from build123d import *

# Parameters (mm, degrees)
ESBO_O1_W                = 49.1
ESBO_O1_H                = 29.84
ESBO_O1_R                = 5.05
RESSALTO_EXTRUS_O1_DEPTH = 1.8
ESBO_O2_W                = 42
ESBO_O2_H                = 29.84
ESBO_O2_R                = 1.35
RESSALTO_EXTRUS_O2_DEPTH = 1.8
RESSALTO_EXTRUS_O3_START = 1.8
ESBO_O3_W                = 42
ESBO_O3_H                = 29.84
ESBO_O3_R                = 1.35
RESSALTO_EXTRUS_O3_DEPTH = 1.8


with BuildPart() as part:
    # Esboço1 → Ressalto-extrusão1 (new body)
    with BuildSketch(Plane.XY):
        Rectangle(ESBO_O1_W, ESBO_O1_H)
        Circle(ESBO_O1_R, mode=Mode.SUBTRACT)
    extrude(amount=RESSALTO_EXTRUS_O1_DEPTH)

    # Esboço2 → Ressalto-extrusão2 (add)
    with BuildSketch(Plane.ZY.offset(24.55)):
        with Locations((21, 0)):
            Rectangle(ESBO_O2_W, ESBO_O2_H)
        with Locations((32, 0)):
            Circle(ESBO_O2_R, mode=Mode.SUBTRACT)
        with Locations((25.05, 7)):
            Circle(ESBO_O2_R, mode=Mode.SUBTRACT)
        with Locations(Location((18, 0, 0), (0, 0, 180))):
            Circle(ESBO_O2_R, mode=Mode.SUBTRACT)
        with Locations(Location((25.05, -7, 0), (0, 0, 180))):
            Circle(ESBO_O2_R, mode=Mode.SUBTRACT)
    extrude(amount=RESSALTO_EXTRUS_O2_DEPTH)

    # Esboço3 → Ressalto-extrusão3 (add)
    with BuildSketch(Plane(origin=(24.55, 0, 0), x_dir=(0, 0, -1), z_dir=(1, 0, 0)).offset(RESSALTO_EXTRUS_O3_START)):
        with Locations((-21, 0)):
            Rectangle(ESBO_O3_W, ESBO_O3_H)
        with Locations(Location((-25.05, 7, 0), (0, 0, 180))):
            Circle(ESBO_O3_R, mode=Mode.SUBTRACT)
        with Locations((-18, 0)):
            Circle(ESBO_O3_R, mode=Mode.SUBTRACT)
        with Locations(Location((-32, 0, 0), (0, 0, 180))):
            Circle(ESBO_O3_R, mode=Mode.SUBTRACT)
        with Locations((-25.05, -7)):
            Circle(ESBO_O3_R, mode=Mode.SUBTRACT)
    extrude(amount=-RESSALTO_EXTRUS_O3_DEPTH)


solid = part.part
Input: part model. Units: mm. Frame: model coordinates. A direction names the side the tool comes from. Coordinates: 2 decimals unless noted, no trailing zeros. Loops run counter-clockwise (first coordinate to the right, second up) from the corner with the lowest first, then second, coordinate; pieces in that order, holes last. Notation, with made-up numbers: (32.25, -39.5) -> (78.25, -39.5) arc R14 ccw to (78.25, -30.5) -> close; hole circle Ø3 at (89.25, 67.25). An arc over 180 degrees is marked (long way). One line per item, written item: value.
(1) Ray query, line 1 along Y through (x, z) = (-25.1, 25.05); line 2 along Y through (x, z) = (25.95, 32); line 3 along X through (y, z) = (-8, 23.5). Return the intervals inside material, ascending.
Answer below:
line 1: y = -14.92 to -8.35, -5.65 to 5.65, 8.35 to 14.92
line 2: y = -14.92 to -1.35, 1.35 to 14.92
line 3: x = -26.35 to -24.55, 24.55 to 26.35
(2) Set-up query: faces 4 (the face through (25, 0, 42)), 5 (the face through (-24.55, 0, 22)). Return all of +Z, -Z, +X, -X, +Y, -Y with unobstructed straight access to the full face (end or side cutting, diameter ignored); none if empty.
Answer below:
face 4: +Z, +X, -X, +Y, -Y
face 5: +Z, +Y, -Y
(3) Cut plane B-B (y = -7). Output: boundary loops of the cut face in (x, z), then the cut area to 3 significant figures.
Answer below:
outline: (-26.35, 0) -> (26.35, 0) -> (26.35, 23.7) -> (24.55, 23.7) -> (24.55, 1.8) -> (-24.55, 1.8) -> (-24.55, 23.7) -> (-26.35, 23.7) -> close; (-26.35, 26.4) -> (-24.55, 26.4) -> (-24.55, 42) -> (-26.35, 42) -> close; (24.55, 26.4) -> (26.35, 26.4) -> (26.35, 42) -> (24.55, 42) -> close
area: 230 mm2
(4) Cut plane A-A (x = 0). Output: boundary loops of the cut face in (y, z), then the cut area to 3 significant figures.
Answer below:
outline: (-14.92, 0) -> (-5.05, 0) -> (-5.05, 1.8) -> (-14.92, 1.8) -> close; (5.05, 0) -> (14.92, 0) -> (14.92, 1.8) -> (5.05, 1.8) -> close
area: 35.5 mm2
(5) Cut plane D-D (y = 0). Output: boundary loops of the cut face in (x, z).
Answer below:
outline: (-26.35, 0) -> (-5.05, 0) -> (-5.05, 1.8) -> (-24.55, 1.8) -> (-24.55, 16.65) -> (-26.35, 16.65) -> close; (-26.35, 19.35) -> (-24.55, 19.35) -> (-24.55, 30.65) -> (-26.35, 30.65) -> close; (-26.35, 33.35) -> (-24.55, 33.35) -> (-24.55, 42) -> (-26.35, 42) -> close; (5.05, 0) -> (26.35, 0) -> (26.35, 16.65) -> (24.55, 16.65) -> (24.55, 1.8) -> (5.05, 1.8) -> close; (24.55, 19.35) -> (26.35, 19.35) -> (26.35, 30.65) -> (24.55, 30.65) -> close; (24.55, 33.35) -> (26.35, 33.35) -> (26.35, 42) -> (24.55, 42) -> close
(6) Pin query (flat end, axial travel): pin 1 Ø3 at (x, y) = (0, -11.5) entering from -Z; pin 2 Ø11.5 at (x, y) = (0, 0) entering from +Z. Return the tip coordinate at first contact, or that it passes through.
Answer below:
pin 1: stops at z = 0
pin 2: stops at z = 1.8
(7) Draft query along X for faces 1 (the face through (-6, 0, 1.8)), 2 (the face through (0, -14.92, 1)), 3 (the face through (-26.35, 0, 21)). Return one class per face: pulls with the +X half, pulls with the -X half, needs draft (parallel to the pull), parting line crosses it, or undercut.
Answer below:
face 1: undercut
face 2: needs draft
face 3: pulls with the -X half
(8) Cut plane C-C (z = 18). Output: boundary loops of the cut face in (x, y).
Answer below:
outline: (-26.35, -14.92) -> (-24.55, -14.92) -> (-24.55, -1.35) -> (-26.35, -1.35) -> close; (-26.35, 1.35) -> (-24.55, 1.35) -> (-24.55, 14.92) -> (-26.35, 14.92) -> close; (24.55, -14.92) -> (26.35, -14.92) -> (26.35, -1.35) -> (24.55, -1.35) -> close; (24.55, 1.35) -> (26.35, 1.35) -> (26.35, 14.92) -> (24.55, 14.92) -> close
